from build123d import *

# Parameters (mm, degrees)
SKETCH1_R           = 3
SKETCH1_R_2         = 1
BOSS_EXTRUDE1_DEPTH = 10
SKETCH2_R           = 4
BOSS_EXTRUDE2_DEPTH = 10
SKETCH3_R           = 4
BOSS_EXTRUDE3_DEPTH = 15
DRAFT1_ANGLE        = 2


with BuildPart() as part:
    # Sketch1 → Boss-Extrude1 (new body)
    with BuildSketch(Plane(origin=(0, 0, 0), x_dir=(1, 0, 0), z_dir=(0, 1, 0))):
        Circle(SKETCH1_R)
        Circle(SKETCH1_R_2, mode=Mode.SUBTRACT)
    extrude(amount=BOSS_EXTRUDE1_DEPTH)

    # Sketch2 → Boss-Extrude2 (add)
    with BuildSketch(Plane(origin=(0, 10, 0), x_dir=(1, 0, 0), z_dir=(0, 1, 0))):
        Circle(SKETCH2_R)
    extrude(amount=BOSS_EXTRUDE2_DEPTH)

    # Sketch3 → Boss-Extrude3 (add)
    with BuildSketch(Plane(origin=(0, 20, 0), x_dir=(1, 0, 0), z_dir=(0, 1, 0))):
        Circle(SKETCH3_R)
    extrude(amount=BOSS_EXTRUDE3_DEPTH)

    # Draft1
    draft1_faces = [part.faces().sort_by_distance(p)[0] for p in [
        (-4, 22.5, 0),
    ]]
    draft(draft1_faces, Plane.ZX.offset(35), DRAFT1_ANGLE)


solid = part.part
Build history of the part. All positions in model axes, mm. A direction names the side the tool comes from. Round coordinates to 2 decimals unless told otherwise and drop trailing zeros. Write each loop counter-clockwise with the first axis right and the second up, starting at its lowest first coordinate (ties: lowest second). Pieces come first, ordered by that corner, then holes. Notation, with made-up numbers: M 12.25,-32 L 26.25,-32 A32 ccw 26.25,-4 Z; hole C 46,24.25 d4. An arc over 180 degrees is marked long. Answer in a Markdown table with one row per item.
1. Mould opens along Z. For faces 1 (the face through (-1, 0, -1)), 2 (the face through (0, 5, 1)), 3 (the face through (-0.963, 22.325, 4.337)) say: +Z half, -Z half, draft (parallel to the pull), parting line (faces both ways), or undercut.
Geometry check:
| item | result |
|---|---|
| face 1 | draft |
| face 2 | undercut |
| face 3 | parting line |
2. Saw through at C-C (y = 7). List the corners of the cut face in (x, z).
Geometry check:
| item | result |
|---|---|
| outline | C 0,0 d6; hole C 0,0 d2 |
3. Saw through at D-D (y = 12). List the corners of the cut face in (x, z), and give its area (3 significant figures).
Geometry check:
| item | result |
|---|---|
| outline | C 0,0 d9.61 |
| area | 72.5 mm2 |
4. Saw through at B-B (x = 0). List the corners of the cut face in (y, z), and give its area (3 significant figures).
Geometry check:
| item | result |
|---|---|
| outline | M 0,-3 L 10,-3 L 10,-4.87 L 35,-4 L 35,4 L 10,4.87 L 10,3 L 0,3 L 0,1 L 10,1 L 10,-1 L 0,-1 Z |
| area | 262 mm2 |
5. Probe L1, parallel to Z at x = 0, y = 6.5; L2, parallel to Y at x = -3.5, z = 1.75. List the from-to ranges inside material, lowest first. Write a range as [from, to].
Geometry check:
| item | result |
|---|---|
| L1 | [-3, -1], [1, 3] |
| L2 | [10, 35] |
6. Which spindle directions (+Z, -Z, +X, -X, +Y, -Y) get a long thin tool onto all of the face, cutting with end or side? Do faces 4 (the face through (0, 35, 0)), 5 (the face through (-3, 5, 0)). Say none if no direction does.
Geometry check:
| item | result |
|---|---|
| face 4 | +Z, -Z, +X, -X, +Y |
| face 5 | -Y |
7. Saw through at A-A (z = 0). List the corners of the cut face in (x, y), and give its area (3 significant figures).
Geometry check:
| item | result |
|---|---|
| outline | M -4.87,10 L -3,10 L -3,0 L -1,0 L -1,10 L 1,10 L 1,0 L 3,0 L 3,10 L 4.87,10 L 4,35 L -4,35 Z |
| area | 262 mm2 |
8. Flat gauge pins, fed straight in: P1, Ø1, axis at x = 3, y = 23.5, coming from the +Z side; P2, Ø5, axis at x = -3.5, y = 19, coming from the -Z side; P3, Ø3, axis at x = -3, y = 12, coming from the +Z side. Where does each tip first touch, or does it go through?
Geometry check:
| item | result |
|---|---|
| P1 | z = 3.62 |
| P2 | z = -4.45 |
| P3 | z = 4.57 |
